Could you check a few things on this drawing? It's one solid part, dimensions in mm from its lowest x, y, z. A direction names the side the tool comes from. Give positions to 0.01 mm unless a question says otherwise; leave off trailing zeros. Loops run counter-clockwise (first coordinate to the right, second up) from the corner with the lowest first, then second, coordinate; pieces in that order, holes last. Notation, with made-up numbers: (-39, -3.5) -> (-30, -3.5) arc R31 cw to (-30, 28.5) -> close; hole circle Ø9 at (-22.75, -35). An arc over 180 degrees is marked (long way). Use CSV: the item, a comma, the result in double quotes.
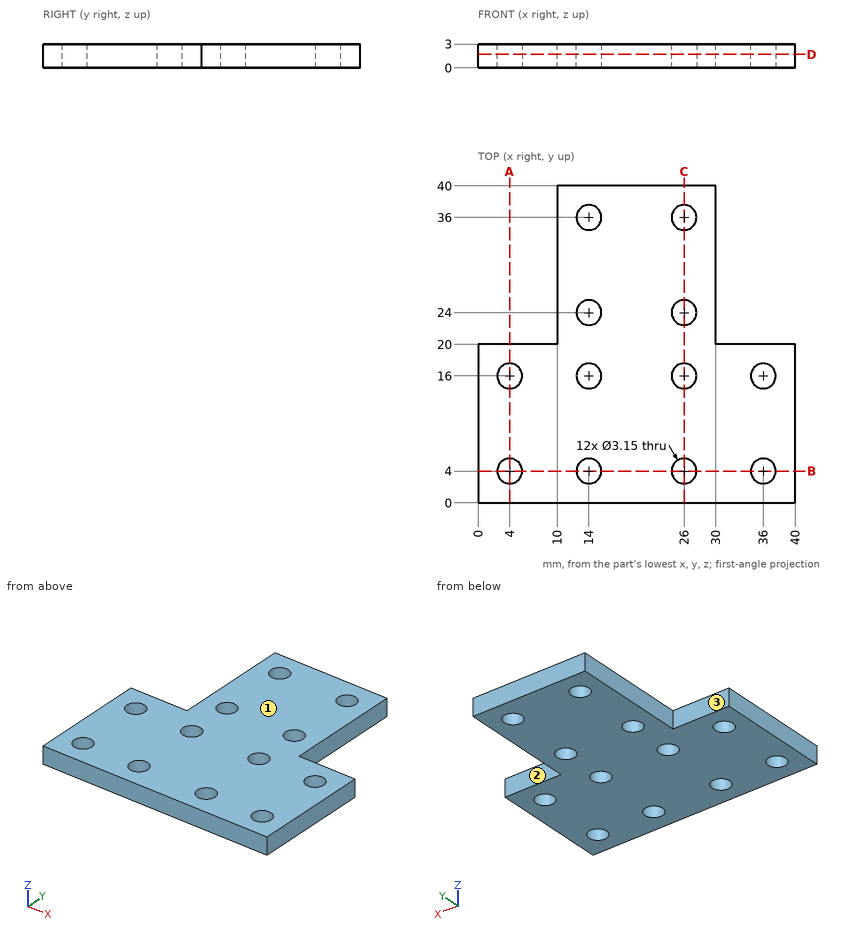
(1) Will these pins go through, and if not, where does the flat tip stop? pin 1 Ø3 at (x, y) = (14, 16) entering from -Z; pin 2 Ø1 at (x, z) = (4.5, 1) entering from +Y; pin 3 Ø0.9 at (y, z) = (29, 1) entering from +X.
Answer sheet:
pin 1,"passes through"
pin 2,"stops at y = 20"
pin 3,"stops at x = 30"
(2) If we section it at D-D, the plane z = 1.7: Give the number of separate pieces and of enclosed holes in the cut face, then the cut area to 3 significant figures.
Answer sheet:
separate pieces,"1"
enclosed holes,"12"
area,"1,110 mm2"
(3) If we section it at C-C, the plane x = 26: Write out the boundary of the cut face in (y, z) (3 decimals).
Answer sheet:
outline,"(0, 0) -> (2.425, 0) -> (2.425, 3) -> (0, 3) -> close; (5.575, 0) -> (14.425, 0) -> (14.425, 3) -> (5.575, 3) -> close; (17.575, 0) -> (22.425, 0) -> (22.425, 3) -> (17.575, 3) -> close; (25.575, 0) -> (34.425, 0) -> (34.425, 3) -> (25.575, 3) -> close; (37.575, 0) -> (40, 0) -> (40, 3) -> (37.575, 3) -> close"
(4) If we section it at A-A, the plane x = 4: Write out the boundary of the cut face in (y, z) (3 decimals), then the cut area to 3 significant figures.
Answer sheet:
outline,"(0, 0) -> (2.425, 0) -> (2.425, 3) -> (0, 3) -> close; (5.575, 0) -> (14.425, 0) -> (14.425, 3) -> (5.575, 3) -> close; (17.575, 0) -> (20, 0) -> (20, 3) -> (17.575, 3) -> close"
area,"41.1 mm2"
(5) If we section it at B-B, the plane y = 4: Write out the boundary of the cut face in (x, z) (3 decimals), then the cut area to 3 significant figures.
Answer sheet:
outline,"(0, 0) -> (2.425, 0) -> (2.425, 3) -> (0, 3) -> close; (5.575, 0) -> (12.425, 0) -> (12.425, 3) -> (5.575, 3) -> close; (15.575, 0) -> (24.425, 0) -> (24.425, 3) -> (15.575, 3) -> close; (27.575, 0) -> (34.425, 0) -> (34.425, 3) -> (27.575, 3) -> close; (37.575, 0) -> (40, 0) -> (40, 3) -> (37.575, 3) -> close"
area,"82.2 mm2"
(6) Which directions (+Z, -Z, +X, -X, +Y, -Y) give clear straight access to the entire face, cutting with the end or side of a thin tool? Please do the marked faces 1, 2 and 3.
Answer sheet:
face 1,"+Z, +X, -X, +Y, -Y"
face 2,"+Z, -Z, +X, +Y"
face 3,"+Z, -Z, -X, +Y"
(7) If I drill on L1, parallel to Y at x = 26, z = 2.2 (3 decimals); L2, parallel to Y at x = 4, z = 2.15 (3 decimals); L3, parallel to Y at x = 13.5, z = 1.55, over which ranges is the centre line in solid material (lowest first)? Write a range as from..to.
Answer sheet:
L1,"y = 0..2.425, 5.575..14.425, 17.575..22.425, 25.575..34.425, 37.575..40"
L2,"y = 0..2.425, 5.575..14.425, 17.575..20"
L3,"y = 0..2.51, 5.49..14.51, 17.49..22.51, 25.49..34.51, 37.49..40"
